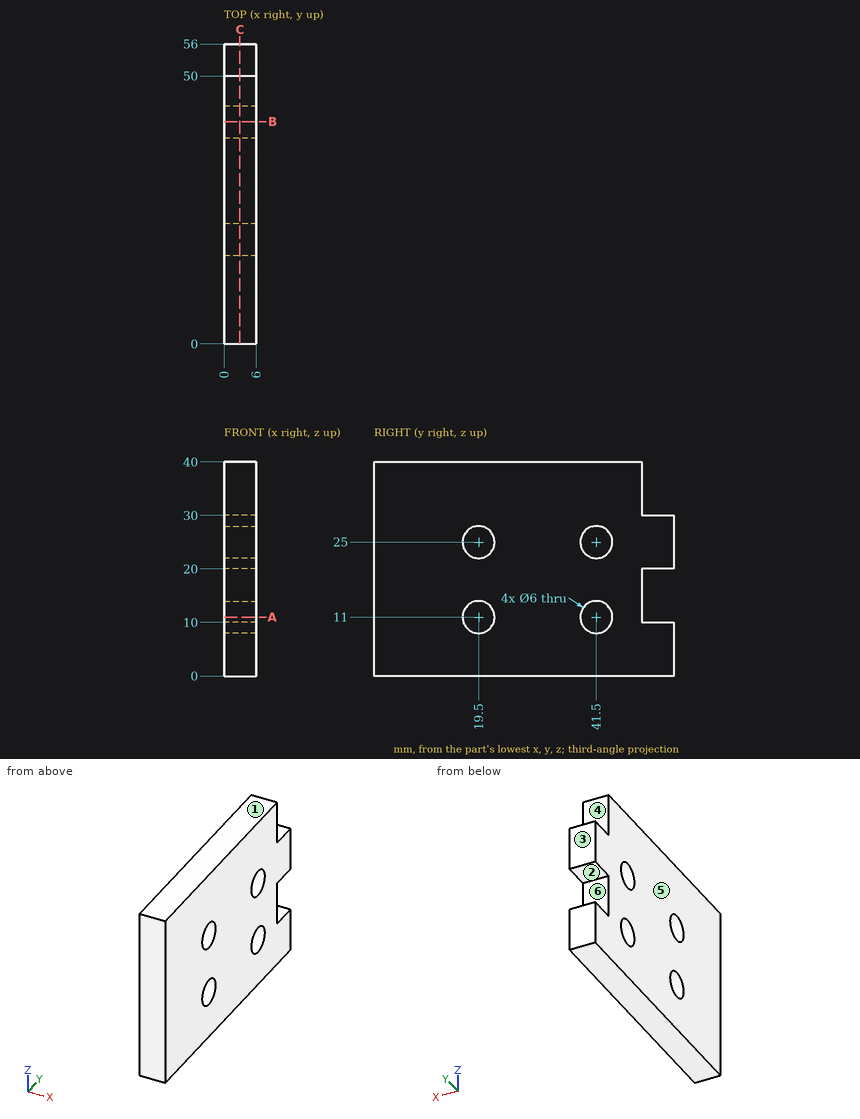
Drawing for the job (mm, zero at the part's lowest x, y, z). A direction names the side the tool comes from. Give positions to 0.01 mm unless a question says otherwise; leave off trailing zeros. Loops run counter-clockwise (first coordinate to the right, second up) from the corner with the lowest first, then second, coordinate; pieces in that order, holes last.
1) 3-axis set-ups, long thin cutter, end or side, ignore diameter. For the marked faces 4, 5 and 6: which of +Z, -Z, +X, -X, +Y, -Y reach the whole face in a straight line?
Values follow:
face 4: +Z, +X, -X, +Y
face 5: +Z, -Z, -X, +Y, -Y
face 6: +X, -X, +Y
2) Two-plate mould, pull along Z, no slides. Class the marked faces 1, 2 and 3: released by +Z, released by -Z, zero draft, split by the parting line, or undercut.
Values follow:
face 1: released by +Z
face 2: undercut
face 3: zero draft
3) Drop flat-ended pins along their axis: P1, Ø3, axis at x = 4, y = 53, coming from the +Z side; P2, Ø3, axis at x = 2.5, z = 34, coming from the +Y side. Give the stop position or say it passes through.
Values follow:
P1: stops at z = 30
P2: stops at y = 50
4) Probe line 1 along Y through (x, z) = (2.6, 11); line 2 along Y through (x, z) = (1.8, 25); line 3 along Z through (x, y) = (4.1, 52). List the from-to ranges inside material, lowest first.
Values follow:
line 1: y = 0 to 16.5, 22.5 to 38.5, 44.5 to 50
line 2: y = 0 to 16.5, 22.5 to 38.5, 44.5 to 56
line 3: z = 0 to 10, 20 to 30
5) Band-saw the part on C-C on x = 2.95. List the corners of the cut face in (y, z).
Values follow:
outline: (0, 0) - (56, 0) - (56, 10) - (50, 10) - (50, 20) - (56, 20) - (56, 30) - (50, 30) - (50, 40) - (0, 40) - close; hole circle Ø6 at (19.5, 11); hole circle Ø6 at (19.5, 25); hole circle Ø6 at (41.5, 11); hole circle Ø6 at (41.5, 25)
6) Band-saw the part on B-B on y = 41.5. List the corners of the cut face in (x, z), then the cut area to 3 significant figures.
Values follow:
outline: (0, 0) - (6, 0) - (6, 8) - (0, 8) - close; (0, 14) - (6, 14) - (6, 22) - (0, 22) - close; (0, 28) - (6, 28) - (6, 40) - (0, 40) - close
area: 168 mm2
7) Band-saw the part on A-A on z = 11. List the corners of the cut face in (x, y), then the cut area to 3 significant figures.
Values follow:
outline: (0, 0) - (6, 0) - (6, 16.5) - (0, 16.5) - close; (0, 22.5) - (6, 22.5) - (6, 38.5) - (0, 38.5) - close; (0, 44.5) - (6, 44.5) - (6, 50) - (0, 50) - close
area: 228 mm2
